```python
from build123d import *

# Parameters (mm, degrees)
ESQUISSE1_R             = 4.5
ESQUISSE1_R_2           = 0.8
BOSS_EXTRU_1_DEPTH      = 3
ESQUISSE2_R             = 4
ENL_V_MAT_EXTRU_1_DEPTH = 10


with BuildPart() as part:
    # Esquisse1 → Boss.-Extru.1 (new body)
    with BuildSketch(Plane.XY):
        with BuildLine():
            Line((1.597834667, 9), (24.597834667, 9))
            ThreePointArc((24.597834667, 9), (33.597834667, 0), (24.597834667, -9))
            Line((24.597834667, -9), (-35.402165333, -9))
            Line((-35.402165333, -9), (-35.402165333, 9))
            Line((-35.402165333, 9), (-16.752165333, 9))
            Line((-16.752165333, 9), (-7.052165333, 9))
            Line((-7.052165333, 9), (1.597834667, 9))
        make_face()
        with Locations((24.597834667, 0)):
            Circle(ESQUISSE1_R, mode=Mode.SUBTRACT)
        with Locations((22.97907079, 7)):
            Circle(ESQUISSE1_R_2, mode=Mode.SUBTRACT)
        with Locations((28.402943221, 6.094386383)):
            Circle(ESQUISSE1_R_2, mode=Mode.SUBTRACT)
        with Locations((31.597834667, 1.618763877)):
            Circle(ESQUISSE1_R_2, mode=Mode.SUBTRACT)
        with Locations((30.69222105, -3.805108554)):
            Circle(ESQUISSE1_R_2, mode=Mode.SUBTRACT)
        with Locations((26.216598544, -7)):
            Circle(ESQUISSE1_R_2, mode=Mode.SUBTRACT)
        with Locations((20.792726113, -6.094386383)):
            Circle(ESQUISSE1_R_2, mode=Mode.SUBTRACT)
        with Locations((17.597834667, -1.618763877)):
            Circle(ESQUISSE1_R_2, mode=Mode.SUBTRACT)
        with Locations((18.503448284, 3.805108554)):
            Circle(ESQUISSE1_R_2, mode=Mode.SUBTRACT)
    extrude(amount=BOSS_EXTRU_1_DEPTH)

    # Esquisse2 → Enlèv. mat.-Extru.1 (cut)
    with BuildSketch(Plane.XY.offset(3)):
        with Locations((-27.402165333, 0)):
            Circle(ESQUISSE2_R)
        with Locations((-10.402165333, 0)):
            Circle(ESQUISSE2_R)
    extrude(amount=-ENL_V_MAT_EXTRU_1_DEPTH, mode=Mode.SUBTRACT)


solid = part.part
```
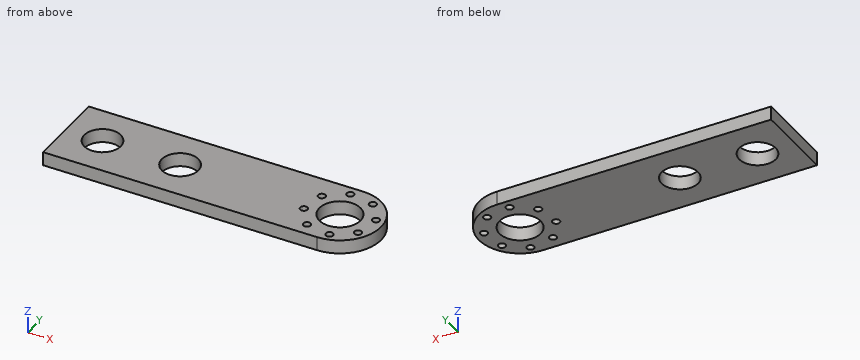
Read the model definition and answer for the solid it produces. Units are mm, in the model's axes. Coordinates: 2 decimals unless noted, no trailing zeros. Write each loop counter-clockwise with the first axis right and the second up, starting at its lowest first coordinate (ties: lowest second). Pieces come first, ordered by that corner, then holes. Notation, with made-up numbers: (25, 2) -> (39, 2) arc R28 ccw to (39, 22) -> close; hole circle Ø1 at (-9.75, 76.25). An arc over 180 degrees is marked (long way). Return JSON: item names as keys, results as strings.
1. Find the intervals of material crossed by line 1 along X through (y, z) = (-2, 1.7); line 2 along Y through (x, z) = (28, 0.4); line 3 along Y through (x, z) = (20.5, 1.7), in increasing order. Write a range as from..to.
Found:
{"line 1": "-35.4..-30.87, -23.94..-13.87, -6.94..16.89, 18.3..20.57, 28.63..33.37", "line 2": "-8.33..-2.95, 2.95..5.4, 6.79..8.33", "line 3": "-9..-6.84, -5.35..-1.86, 1.86..9"}
2. This flat-tipped pin is pushed along its axis until it touches: P1, Ø6.5, axis at x = -27.4, y = 0, coming from the +Z side. Where does it stop, or does it pass through?
Found:
{"P1": "through"}
3. A cutting plane is placed at A-A (y = 0). Determine the outline of the cut face in (x, z).
Found:
{"outline": "(-35.4, 0) -> (-31.4, 0) -> (-31.4, 3) -> (-35.4, 3) -> close; (-23.4, 0) -> (-14.4, 0) -> (-14.4, 3) -> (-23.4, 3) -> close; (-6.4, 0) -> (20.1, 0) -> (20.1, 3) -> (-6.4, 3) -> close; (29.1, 0) -> (33.6, 0) -> (33.6, 3) -> (29.1, 3) -> close"}
4. A cutting plane is placed at C-C (x = -7). Determine the outline of the cut face in (y, z), and give its area (3 significant figures).
Found:
{"outline": "(-9, 0) -> (-2.1, 0) -> (-2.1, 3) -> (-9, 3) -> close; (2.1, 0) -> (9, 0) -> (9, 3) -> (2.1, 3) -> close", "area": "41.4 mm2"}
5. A cutting plane is placed at B-B (z = 2.1). Give the number of separate pieces and of enclosed holes in the cut face, and give its area (3 significant figures).
Found:
{"separate pieces": "1", "enclosed holes": "11", "area": "1,030 mm2"}
